Build history of the part. All positions in model axes, mm. A direction names the side the tool comes from. Coordinates: 2 decimals unless noted, no trailing zeros. Order: outer loops, then holes, each group sorted by start corner. A loop starts at its lowest first (then second) coordinate and runs counter-clockwise, first axis right, second up. Notation, with made-up numbers: (32.5, 62) - (55.5, 62) arc R18 ccw to (55.5, 71) - close; hole circle Ø8 at (67, -16). An arc over 180 degrees is marked (long way). Write each question's results on one line, items separated by ' | '.
from build123d import *

# Parameters (mm, degrees)
BOSS_EXTRUDE1_DEPTH = 10
SKETCH2_W           = 14
SKETCH2_H           = 7
SKETCH2_R           = 1.75
CUT_EXTRUDE1_DEPTH  = 8
SKETCH3_W           = 1
SKETCH3_H           = 2
BOSS_EXTRUDE2_DEPTH = 14
SKETCH4_W           = 1.5
SKETCH4_H           = 8
BOSS_EXTRUDE3_DEPTH = 5.5
SKETCH5_W           = 17
SKETCH5_H           = 10
SKETCH5_W_2         = 6.5
SKETCH5_H_2         = 8
CUT_EXTRUDE2_DEPTH  = 1
FILLET2_R           = 1


with BuildPart() as part:
    # Sketch1 → Boss-Extrude1 (new body)
    with BuildSketch(Plane(origin=(0, 0, 0), x_dir=(1, 0, 0), z_dir=(0, 1, 0))):
        with BuildLine():
            Line((-7.5, -5), (7.5, -5))
            ThreePointArc((7.5, -5), (8.207106781, -4.707106781), (8.5, -4))
            Line((8.5, -4), (8.5, 4))
            ThreePointArc((8.5, 4), (8.207106781, 4.707106781), (7.5, 5))
            Line((7.5, 5), (-7.5, 5))
            ThreePointArc((-7.5, 5), (-8.207106781, 4.707106781), (-8.5, 4))
            Line((-8.5, 4), (-8.5, -4))
            ThreePointArc((-8.5, -4), (-8.207106781, -4.707106781), (-7.5, -5))
        make_face()
    extrude(amount=BOSS_EXTRUDE1_DEPTH)

    # Sketch2 → Cut-Extrude1 (cut)
    with BuildSketch(Plane(origin=(0, 0, 0), x_dir=(1, 0, 0), z_dir=(0, 1, 0))):
        Rectangle(SKETCH2_W, SKETCH2_H)
        with Locations(Location((0, 0, 0), (0, 0, 270))):
            Circle(SKETCH2_R, mode=Mode.SUBTRACT)
    extrude(amount=CUT_EXTRUDE1_DEPTH, mode=Mode.SUBTRACT)

    # Sketch3 → Boss-Extrude2 (add)
    with BuildSketch(Plane(origin=(-7, 0, 0), x_dir=(0, 0, -1), z_dir=(1, 0, 0))):
        with Locations((0, 1)):
            Rectangle(SKETCH3_W, SKETCH3_H)
    extrude(amount=BOSS_EXTRUDE2_DEPTH)

    # Sketch4 → Boss-Extrude3 (add)
    with BuildSketch(Plane.XZ):
        with Locations((9.25, 0)):
            Rectangle(SKETCH4_W, SKETCH4_H)
    extrude(amount=-BOSS_EXTRUDE3_DEPTH)

    # Sketch5 → Cut-Extrude2 (cut)
    with BuildSketch(Plane(origin=(0, 10, 0), x_dir=(1, 0, 0), z_dir=(0, 1, 0))):
        Rectangle(SKETCH5_W, SKETCH5_H)
        with Locations((-4.25, 0)):
            Rectangle(SKETCH5_W_2, SKETCH5_H_2, mode=Mode.SUBTRACT)
        with Locations((4.25, 0)):
            Rectangle(SKETCH5_W_2, SKETCH5_H_2, mode=Mode.SUBTRACT)
    extrude(amount=-CUT_EXTRUDE2_DEPTH, mode=Mode.SUBTRACT)

    # Fillet2
    fillet2_edges = [part.edges().sort_by_distance(p)[0] for p in [
        (-7.5, 9.5, -4),
        (-1, 9.5, -4),
        (-1, 9.5, 4),
        (-7.5, 9.5, 4),
        (1, 9.5, -4),
        (7.5, 9.5, -4),
        (7.5, 9.5, 4),
        (1, 9.5, 4),
        (1, 9, 0),
        (4.25, 9, 4),
        (7.5, 9, 0),
        (4.25, 9, -4),
        (-7.5, 9, 0),
        (-4.25, 9, 4),
        (-1, 9, 0),
        (-4.25, 9, -4),
    ]]
    fillet(fillet2_edges, radius=FILLET2_R - 0.0001)  # a hair under: the kernel refuses the full size


solid = part.part
1. Band-saw the part on D-D on z = 0. Give the number of separate pieces and of enclosed holes in the cut face, then the cut area to 3 significant figures.
Solved:
separate pieces: 1 | enclosed holes: 2 | area: 112 mm2
2. Band-saw the part on C-C on y = 8.5. Give the cut face in (x, z), then the cut area to 3 significant figures.
Solved:
outline: (-8.5, -4) arc R1 ccw to (-7.5, -5) - (7.5, -5) arc R1 ccw to (8.5, -4) - (8.5, 4) arc R1 ccw to (7.5, 5) - (-7.5, 5) arc R1 ccw to (-8.5, 4) - close | area: 169 mm2
3. Drop flat-ended pins along their axis: pin 1 Ø1 at (y, z) = (6.5, 0.5) entering from +X; pin 2 Ø1.2 at (x, z) = (9, 1) entering from +Y (3 decimals). Give the stop position or say it passes through.
Solved:
pin 1: stops at x = 8.5 | pin 2: stops at y = 9.005
4. Probe line 1 (Z direction, x = 6, y = 1.75); line 2 (Z direction, x = 1, y = 1); line 3 (Z direction, x = 6, y = 5.5). List the from-to ranges inside material, lowest first.
Solved:
line 1: z = -5 to -3.5, -0.5 to 0.5, 3.5 to 5 | line 2: z = -5 to -3.5, -1.44 to 1.44, 3.5 to 5 | line 3: z = -5 to -3.5, 3.5 to 5
5. Two-plate mould, pull along Y, no slides. Class faces 6 (the face through (1, 0, 0)), 7 (the face through (9, 5.5, 0)), 8 (the face through (-4, 2, 0)), 9 (the face through (4, 1, -0.5)): +Y half, -Y half, draft (parallel to the pull), parting line (faces both ways), or undercut.
Solved:
face 6: -Y half | face 7: +Y half | face 8: undercut | face 9: draft
6. Band-saw the part on A-A on y = 2.25. Give the cut face in (x, z), then the cut area to 3 significant figures.
Solved:
outline: (-8.5, -4) arc R1 ccw to (-7.5, -5) - (7.5, -5) arc R1 ccw to (8.5, -4) - (10, -4) - (10, 4) - (8.5, 4) arc R1 ccw to (7.5, 5) - (-7.5, 5) arc R1 ccw to (-8.5, 4) - close; circle Ø3.5 at (0, 0); hole (-7, -3.5) - (7, -3.5) - (7, 3.5) - (-7, 3.5) - close | area: 92.8 mm2
7. Tool access for faces 1 (the face through (-7.801, 9.285, -0.042)), 2 (the face through (8.5, 7, 0)), 3 (the face through (-4, 1, -0.5)), 4 (the face through (-8.215, 4.437, 4.699)), 5 (the face through (9, 3, 4)): list every direction of +Z, -Z, +X, -X, +Y, -Y with a clear straight run to the whole face (end or side of a thin tool).
Solved:
face 1: +Z, -Z, -X, +Y | face 2: +Z, -Z, +X, +Y | face 3: -Y | face 4: +Z, -X, +Y, -Y | face 5: +Z, +X, +Y, -Y
